from build123d import *

# Parameters (mm, degrees)
SALIENTE_EXTRUIR1_DEPTH = 16
CROQUIS3_R              = 30.5
CORTAR_EXTRUIR3_DEPTH   = 135.093251135
CROQUIS4_R              = 35.5
CORTAR_EXTRUIR4_DEPTH   = 12
SALIENTE_EXTRUIR2_DEPTH = 49
CROQUIS6_W              = 80
CROQUIS6_H              = 62
SALIENTE_EXTRUIR4_DEPTH = 4
CROQUIS8_W              = 10
CROQUIS8_H              = 34.666666667
CORTAR_EXTRUIR6_DEPTH   = 229.089894559
CROQUIS9_R              = 3
CORTAR_EXTRUIR7_DEPTH   = 189.148877222
REDONDEO1_R             = 5
CROQUIS10_R             = 2.5
CORTAR_EXTRUIR8_DEPTH   = 156.32224567
CROQUIS11_R             = 2.5
CORTAR_EXTRUIR9_DEPTH   = 10


with BuildPart() as part:
    # Croquis2 → Saliente-Extruir1 (new body)
    with BuildSketch(Plane.XY):
        with BuildLine():
            Line((-65, 110), (65, 110))
            ThreePointArc((65, 110), (72.071067812, 107.071067812), (75, 100))
            Line((75, 100), (75, -100))
            ThreePointArc((75, -100), (72.071067812, -107.071067812), (65, -110))
            Line((65, -110), (-65, -110))
            ThreePointArc((-65, -110), (-72.071067812, -107.071067812), (-75, -100))
            Line((-75, -100), (-75, 100))
            ThreePointArc((-75, 100), (-72.071067812, 107.071067812), (-65, 110))
        make_face()
    extrude(amount=SALIENTE_EXTRUIR1_DEPTH)

    # Croquis3 → Cortar-Extruir3 (cut, through all)
    with BuildSketch(Plane.XY.offset(16)):
        with Locations((0, 50)):
            Circle(CROQUIS3_R)
    extrude(amount=-CORTAR_EXTRUIR3_DEPTH, mode=Mode.SUBTRACT)

    # Croquis4 → Cortar-Extruir4 (cut)
    with BuildSketch(Plane.XY.offset(16)):
        with Locations((0, 50)):
            Circle(CROQUIS4_R)
    extrude(amount=-CORTAR_EXTRUIR4_DEPTH, mode=Mode.SUBTRACT)

    # Croquis5 → Saliente-Extruir2 (add)
    with BuildSketch(Plane(origin=(0, 0, 0), x_dir=(-1, 0, 0), z_dir=(0, 0, -1))):
        Polygon((-55, 83), (-55, 10), (-51, 10), (-51, 79), (-51, 86), (-44, 86), (44, 86), (51, 86), (51, 79), (51, 10), (55, 10), (55, 83), (55, 90), (48, 90), (-48, 90), (-55, 90), align=None)
    extrude(amount=SALIENTE_EXTRUIR2_DEPTH)

    # Croquis6 → Saliente-Extruir4 (add)
    with BuildSketch(Plane(origin=(0, 90, 0), x_dir=(1, 0, 0), z_dir=(0, 1, 0))):
        with Locations((0, 49)):
            Rectangle(CROQUIS6_W, CROQUIS6_H)
    extrude(amount=-SALIENTE_EXTRUIR4_DEPTH)

    # Croquis8 → Cortar-Extruir6 (cut, through all)
    with BuildSketch(Plane(origin=(0, 90, 0), x_dir=(1, 0, 0), z_dir=(0, 1, 0))):
        with Locations((-45, 40.333333334)):
            Rectangle(CROQUIS8_W, CROQUIS8_H)
        with Locations((45, 40.333333334)):
            Rectangle(CROQUIS8_W, CROQUIS8_H)
    extrude(amount=-CORTAR_EXTRUIR6_DEPTH, mode=Mode.SUBTRACT)

    # Croquis9 → Cortar-Extruir7 (cut, through all)
    with BuildSketch(Plane(origin=(55, 0, 0), x_dir=(0, 0, -1), z_dir=(1, 0, 0))):
        with Locations((38, 70)):
            Circle(CROQUIS9_R)
    extrude(amount=-CORTAR_EXTRUIR7_DEPTH, mode=Mode.SUBTRACT)

    # Redondeo1
    redondeo1_edges = [part.edges().sort_by_distance(p)[0] for p in [
        (-51, 86, -24.5),
        (51, 86, -24.5),
        (55, 90, -24.5),
        (-55, 90, -24.5),
    ]]
    fillet(redondeo1_edges, radius=REDONDEO1_R - 0.0001)  # a hair under: the kernel refuses the full size

    # Croquis10 → Cortar-Extruir8 (cut, through all)
    with BuildSketch(Plane(origin=(0, 0, 0), x_dir=(-1, 0, 0), z_dir=(0, 0, -1))):
        with Locations((-42, 50.158024554)):
            Circle(CROQUIS10_R)
        with Locations((41.5, 50.158024554)):
            Circle(CROQUIS10_R)
    extrude(amount=-CORTAR_EXTRUIR8_DEPTH, mode=Mode.SUBTRACT)

    # Croquis11 → Cortar-Extruir9 (cut)
    with BuildSketch(Plane.XZ.offset(-86)):
        with Locations(Location((32.851728302, -29, 0), (0, 0, 270))):
            Circle(CROQUIS11_R)
        with Locations(Location((32.851728302, -69, 0), (0, 0, 270))):
            Circle(CROQUIS11_R)
        with Locations(Location((-27.516343247, -69, 0), (0, 0, 270))):
            Circle(CROQUIS11_R)
        with Locations(Location((-27.516343247, -29, 0), (0, 0, 270))):
            Circle(CROQUIS11_R)
    extrude(amount=-CORTAR_EXTRUIR9_DEPTH, mode=Mode.SUBTRACT)


solid = part.part
Model file for the job. Use its own axes, mm. A direction names the side the tool comes from. Give positions to 0.01 mm unless a question says otherwise; leave off trailing zeros. Order: outer loops, then holes, each group sorted by start corner. A loop starts at its lowest first (then second) coordinate and runs counter-clockwise, first axis right, second up. Notation, with made-up numbers: (-6, 3) - (39, 3) arc R7 cw to (39, 14) - close; hole circle Ø10 at (25, 68). An arc over 180 degrees is marked (long way). Write item = value, one per line. Start each with the question number.
1. Which spindle directions (+Z, -Z, +X, -X, +Y, -Y) get a long thin tool onto all of the face, cutting with end or side? Do faces 5 (the flat face through (-1, 90, -39)), 6 (the flat face through (1, 86, -39)), 7 (the flat face through (55, 48, -24)), 8 (the flat face through (-53, 51, -49)). Say none if no direction does.
2. Two-plate mould, pull along X, no slides. Class faces 1 (the cylindrical face through (-22.48, 70.613, 2.028)), 2 (the flat face through (1, 2, 16)), 3 (the cylindrical face through (72.15, -106.99, 7.89)), 4 (the cylindrical face through (39.69, 49.2, 7.89)): pulls with the +X half, pulls with the -X half, needs draft (parallel to the pull), parting line crosses it, or undercut.
3. Probe line 1 along Y through (x, z) = (0, 3.2); line 2 along X through (y, z) = (89, -29); line 3 along X through (y, z) = (25, -47). List the from-to ranges inside material, lowest first.
4. Cut at D-D, the plane y = 70. List the corners of the cut face in (x, z).
5. Cut at C-C, the plane z = -18. List the corners of the cut face in (x, y), and give its area (3 significant figures).
6. Cut at B-B, the plane x = 0. List the corners of the cut face in (y, z).
7. Drop flat-ended pins along their axis: P1, Ø5, axis at x = 35, z = -45.5, coming from the -Y side; P2, Ø4.5, axis at y = 88.5, z = -42, coming from the +X side; P3, Ø1, axis at x = -53.5, z = -7.5, coming from the +Y side; P4, Ø3, axis at x = 32.85, z = -29, coming from the +Y side. Give the stop position or say it passes through.
8. Cut at A-A, the plane z = -29. State how many separate pieces and enclosed holes the cut face has, and give its area (3 significant figures).
Taken from the geometry:
q1.face_5 = -Z, +X, -X, +Y
q1.face_6 = -Z, -Y
q1.face_7 = -Z, +X, +Y, -Y
q1.face_8 = -Z, -X, +Y, -Y
q2.face_1 = undercut
q2.face_2 = needs draft
q2.face_3 = pulls with the +X half
q2.face_4 = undercut
q3.line_1 = -110 to 19.5, 80.5 to 110
q3.line_2 = -53 to -50, -40 to -30.02, -25.02 to 30.35, 35.35 to 40, 50 to 53
q3.line_3 = -55 to -51, 51 to 55
q4.outline = (-75, 0) - (-55, 0) - (-55, -35) - (-51, -35) - (-51, 0) - (-23.03, 0) - (-23.03, 4) - (-29.33, 4) - (-29.33, 16) - (-75, 16) - close; (-55, -49) - (-51, -49) - (-51, -41) - (-55, -41) - close; (23.03, 0) - (51, 0) - (51, -35) - (55, -35) - (55, 0) - (75, 0) - (75, 16) - (29.33, 16) - (29.33, 4) - (23.03, 4) - close; (51, -49) - (55, -49) - (55, -41) - (51, -41) - close
q5.outline = (-55, 10) - (-51, 10) - (-51, 81) arc R5 cw to (-46, 86) - (46, 86) arc R5 cw to (51, 81) - (51, 10) - (55, 10) - (55, 85) arc R5 ccw to (50, 90) - (-50, 90) arc R5 ccw to (-55, 85) - close
q5.area = 1,050 mm²
q6.outline = (-110, 0) - (19.5, 0) - (19.5, 4) - (14.5, 4) - (14.5, 16) - (-110, 16) - close; (80.5, 0) - (86, 0) - (86, -80) - (90, -80) - (90, 0) - (110, 0) - (110, 16) - (85.5, 16) - (85.5, 4) - (80.5, 4) - close
q7.P1 = 86
q7.P2 = 54.84
q7.P3 = 89
q7.P4 = through
q8.separate_pieces = 5
q8.enclosed_holes = 0
q8.area = 923 mm²
